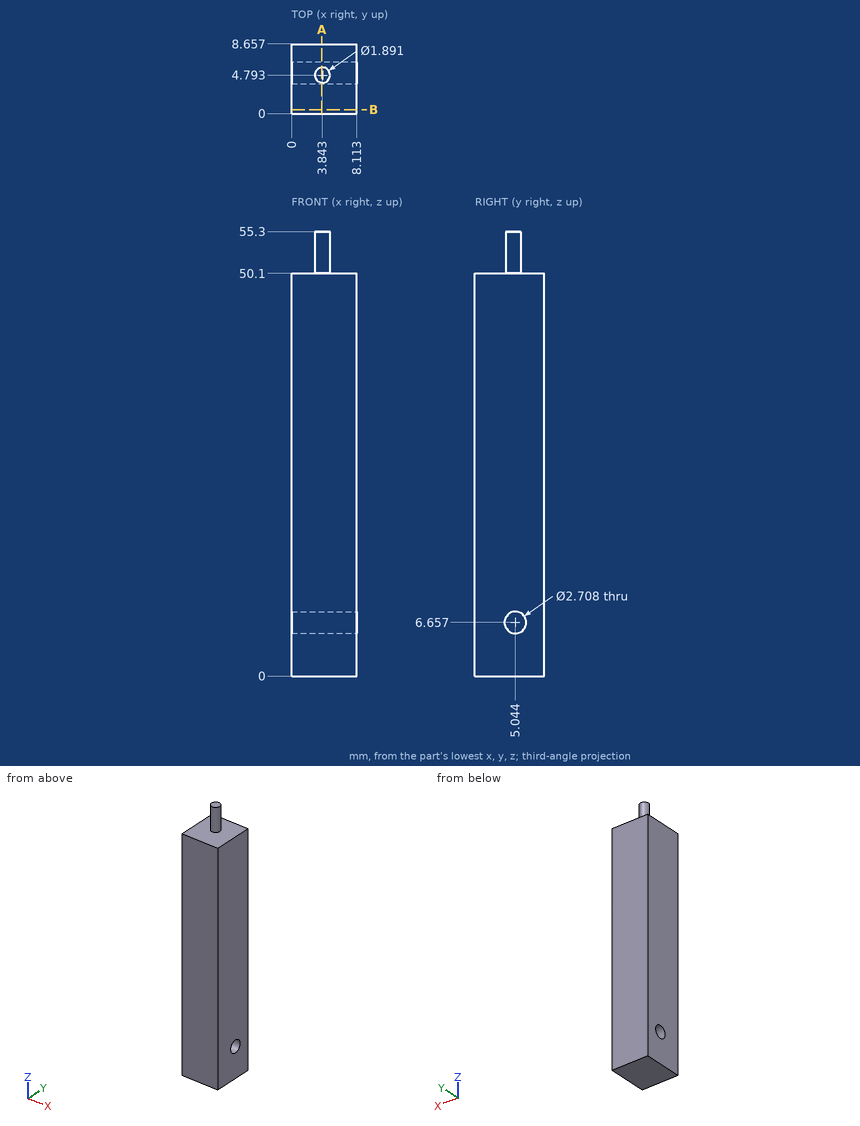
Study the drawing (mm; zero at the part's minimum x, y, z) and answer. Coordinates: 2 decimals unless noted, no trailing zeros. Write each loop counter-clockwise with the first axis right and the second up, starting at its lowest first coordinate (ties: lowest second). Pieces come first, ordered by that corner, then holes. Notation, with made-up numbers: (40, -39.75) - (59, -39.75) arc R12 ccw to (59, -34.75) - close; hole circle Ø7 at (52, 29). An arc over 180 degrees is marked (long way). Answer as a JSON object with one key per item and string values. Group by question number.
1. A cutting plane is placed at B-B (y = 0.5). Determine the outline of the cut face in (x, z).
2. A cutting plane is placed at A-A (x = 3.75). Determine the outline of the cut face in (y, z).
3. Consider L1, parallel to Z at x = 2, y = 5; L2, parallel to Z at x = 1.25, y = 0.75; L3, parallel to Z at x = 1.25, y = 4.5. Determine where each line is inside the solid, lowest interval first. Write a range as [from, to].
4. This flat-tipped pin is pushed along its axis until it touches: P1, Ø1.5, axis at x = 5.5, y = 6.5, coming from the +Z side. Where does it stop, or does it pass through?
Worked out:
{
 "1": {"outline": "(0, 0) - (8.11, 0) - (8.11, 50.1) - (0, 50.1) - close"},
 "2": {"outline": "(0, 0) - (8.66, 0) - (8.66, 50.1) - (5.73, 50.1) - (5.73, 55.3) - (3.85, 55.3) - (3.85, 50.1) - (0, 50.1) - close; hole circle Ø2.71 at (5.04, 6.66)"},
 "3": {"L1": "z = [0, 5.3], [8.01, 50.1]", "L2": "z = [0, 50.1]", "L3": "z = [0, 5.42], [7.9, 50.1]"},
 "4": {"P1": "stops at z = 50.1"}
}
